Design review of the part built by this model. Coordinates are the model's own, in mm. Coordinates: 2 decimals unless noted, no trailing zeros. Write each loop counter-clockwise with the first axis right and the second up, starting at its lowest first coordinate (ties: lowest second). Pieces come first, ordered by that corner, then holes. Notation, with made-up numbers: (14, 35.5) -> (56, 35.5) arc R35 ccw to (56, 71.5) -> close; hole circle Ø3 at (2, 60). An arc over 180 degrees is marked (long way). Answer in a Markdown table with one row per item. Add a question column.
Item 1: Take a section at B-B, the plane z = 0. Write out the cut boundary in (x, y), and give its area (3 significant figures).
Item 2: Take a section at D-D, the plane x = -28.5. Write out the cut boundary in (y, z), and give its area (3 significant figures).
Item 3: Take a section at A-A, the plane x = 0. Write out the cut boundary in (y, z).
Item 4: Take a section at C-C, the plane z = 28. Write out the cut boundary in (x, y) (3 decimals).
Item 5: Draft analysis for pull direction X (two halves, no side actions). For faces 1 (the face through (25.055, 1.521, 25.009)), 2 (the face through (1, 0, 8)), state which applies: released by +X, released by -X, zero draft, split by the parting line, or undercut.
Item 6: To check wall thickness, follow line 1 (X direction, y = 1.6, z = 0); line 2 (Z direction, x = 24.5, y = 2.2); line 3 (X direction, y = 2.4, z = 9). State the ranges of each line that lie inside material, in increasing order.
Item 7: Clearance check with flat-ended pins moving along their axes: P1, Ø0.9, axis at x = -30.5, y = 2, coming from the +Z side; P2, Ø0.9, axis at x = 31, y = 1, coming from the +Z side; P3, Ø1.5, axis at y = 2, z = 25, coming from the +X side. State where each tip first meets the part, or that it passes through.
from build123d import *

# Parameters (mm, degrees)
SKETCH1_R           = 36.5
BOSS_EXTRUDE1_DEPTH = 3
SKETCH2_R           = 3.85
CUT_EXTRUDE1_DEPTH  = 52.705899083
SKETCH3_W           = 4.631754054
SKETCH3_H           = 8.712386095
CUT_EXTRUDE2_DEPTH  = 52.705899083
CIRPATTERN1_COUNT   = 24


with BuildPart() as part:
    # Sketch1 → Boss-Extrude1 (new body)
    with BuildSketch(Plane(origin=(0, 0, 0), x_dir=(1, 0, 0), z_dir=(0, 1, 0))):
        with Locations(Location((0, 0, 0), (0, 0, 270))):
            Circle(SKETCH1_R)
    extrude(amount=BOSS_EXTRUDE1_DEPTH)

    # Sketch2 → Cut-Extrude1 (cut, through all)
    with BuildSketch(Plane(origin=(0, 3, 0), x_dir=(1, 0, 0), z_dir=(0, 1, 0))):
        with Locations(Location((0, 0, 0), (0, 0, 270))):
            Circle(SKETCH2_R)
    extrude(amount=-CUT_EXTRUDE1_DEPTH, mode=Mode.SUBTRACT)

    # Sketch3 → Cut-Extrude2 (cut, through all)
    with BuildSketch(Plane(origin=(0, 3, 0), x_dir=(1, 0, 0), z_dir=(0, 1, 0))):
        with Locations((0, 31.044114287)):
            Rectangle(SKETCH3_W, SKETCH3_H)
    cut_extrude2 = extrude(amount=-CUT_EXTRUDE2_DEPTH, mode=Mode.SUBTRACT)

    # CirPattern1: Cut-Extrude2 ×24 about axis
    cirpattern1_axis = Axis((0, 0, 0), (0, 1, 0))
    for i in range(1, CIRPATTERN1_COUNT):
        add(cut_extrude2.rotate(cirpattern1_axis, i * 360 / CIRPATTERN1_COUNT), mode=Mode.SUBTRACT)


solid = part.part
Answers:
| question | item | result |
|---|---|---|
| 1 | outline | (-36.5, 0) -> (-35.4, 0) -> (-35.4, 3) -> (-36.5, 3) -> close; (-26.69, 0) -> (-3.85, 0) -> (-3.85, 3) -> (-26.69, 3) -> close; (3.85, 0) -> (26.69, 0) -> (26.69, 3) -> (3.85, 3) -> close; (35.4, 0) -> (36.5, 0) -> (36.5, 3) -> (35.4, 3) -> close |
| 1 | area | 144 mm^2 |
| 2 | outline | (0, -22.8) -> (3, -22.8) -> (3, -19.13) -> (0, -19.13) -> close; (0, -13.78) -> (3, -13.78) -> (3, -10.03) -> (0, -10.03) -> close; (0, -5.24) -> (3, -5.24) -> (3, -2.32) -> (0, -2.32) -> close; (0, 2.32) -> (3, 2.32) -> (3, 5.24) -> (0, 5.24) -> close; (0, 10.03) -> (3, 10.03) -> (3, 13.78) -> (0, 13.78) -> close; (0, 19.13) -> (3, 19.13) -> (3, 22.8) -> (0, 22.8) -> close |
| 2 | area | 62.1 mm^2 |
| 3 | outline | (0, -36.5) -> (3, -36.5) -> (3, -35.4) -> (0, -35.4) -> close; (0, -26.69) -> (3, -26.69) -> (3, -3.85) -> (0, -3.85) -> close; (0, 3.85) -> (3, 3.85) -> (3, 26.69) -> (0, 26.69) -> close; (0, 35.4) -> (3, 35.4) -> (3, 36.5) -> (0, 36.5) -> close |
| 4 | outline | (-23.415, 0) -> (-18.84, 0) -> (-18.84, 3) -> (-23.415, 3) -> close; (-13.492, 0) -> (-9.9, 0) -> (-9.9, 3) -> (-13.492, 3) -> close; (-5.105, 0) -> (-2.316, 0) -> (-2.316, 3) -> (-5.105, 3) -> close; (2.316, 0) -> (5.105, 0) -> (5.105, 3) -> (2.316, 3) -> close; (9.9, 0) -> (13.492, 0) -> (13.492, 3) -> (9.9, 3) -> close; (18.84, 0) -> (23.415, 0) -> (23.415, 3) -> (18.84, 3) -> close |
| 5 | face 1 | undercut |
| 5 | face 2 | zero draft |
| 6 | line 1 | x = -36.5 to -35.4, -26.69 to -3.85, 3.85 to 26.69, 35.4 to 36.5 |
| 6 | line 2 | z = -27.06 to -25.56, -21.22 to -16.82, -11.47 to 11.47, 16.82 to 21.22, 25.56 to 27.06 |
| 6 | line 3 | x = -35.37 to -34.24, -25.22 to 25.22, 34.24 to 35.37 |
| 7 | P1 | stops at z = 20.72 |
| 7 | P2 | stops at z = 19.97 |
| 7 | P3 | stops at x = 27.28 |
